Geometry: final body of the model. Coordinates: model frame, mm. Face numbers are marked on the shaded views. A direction names the side the tool comes from. Give positions to 0.01 mm unless a question says otherwise; leave off trailing zeros. Order: outer loops, then holes, each group sorted by start corner. A loop starts at its lowest first (then second) coordinate and runs counter-clockwise, first axis right, second up. Notation, with made-up numbers: M 10.25,37.5 L 20.25,37.5 A16 cw 20.25,41.5 Z; hole C 53.25,-34 d6. An arc over 180 degrees is marked long. Use CSV: the item, a comma, the result in double quotes.
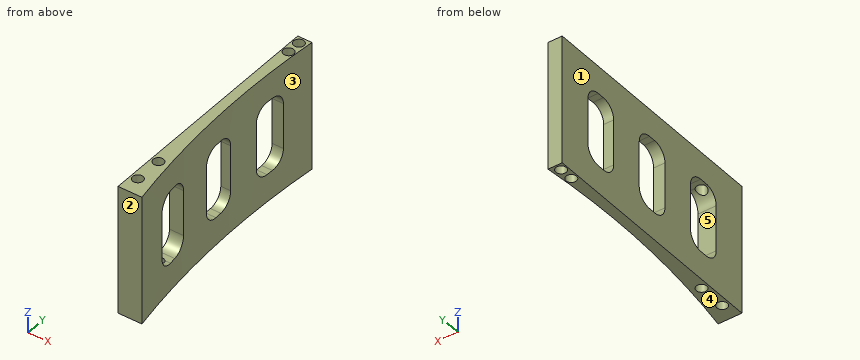
```python
from build123d import *

# Parameters (mm, degrees)
RESSALTO_EXTRUS_O1_DEPTH = 37.2
FILETE3_R                = 10
FILETE4_R                = 10
ESBO_O3_W                = 64.493903811
ESBO_O3_H                = 22.028162523
CORTE_EXTRUS_O2_DEPTH    = 126.622328301
ESBO_O4_W                = 56.697594262
ESBO_O4_H                = 123.119514717
CORTE_EXTRUS_O6_DEPTH    = 126.622328159
ESBO_O7_W                = 25.761955102
ESBO_O7_H                = 34.830585193
CORTE_EXTRUS_O7_DEPTH    = 125.245881598
CORTE_EXTRUS_O8_DEPTH    = 90.772656751
ESBO_O9_R                = 1.5
CORTE_EXTRUS_O9_DEPTH    = 92.227960203


with BuildPart() as part:
    # Esboço1 → Ressalto-extrusão1 (new body)
    with BuildSketch(Plane.XY):
        with BuildLine():
            ThreePointArc((-10, 0), (0, -10), (10, 0))
            Line((10, 0), (20, 0))
            ThreePointArc((20, 0), (14.071698091, 40.495175194), (14.829943665, 81.414963086))
            ThreePointArc((14.829943665, 81.414963086), (11.193742071, 116.066691762), (-16.576524471, 95.024435265))
            Line((-16.576524471, 95.024435265), (-16.487894969, 94.437265709))
            Line((-16.487894969, 94.437265709), (-16.369382775, 93.652123615))
            ThreePointArc((-16.369382775, 93.652123615), (-13.756795166, 46.654405302), (-20, 0))
            Line((-20, 0), (-10, 0))
        make_face()
    extrude(amount=RESSALTO_EXTRUS_O1_DEPTH)

    # Filete3
    # the kernel refuses this fillet: 10 mm, written as the material it takes off along each edge
    with BuildSketch(Plane(origin=(20, 0, -29.463728433), x_dir=(-0.20232831186330175, 0.9793177493635794, 0), z_dir=(0, 0, 1))) as filete3_piece_1:
        with BuildLine():
            CenterArc((12.021201201, 9.997221658), FILETE3_R, 181.169168083, 87.480189)
            Line((2.023283119, 9.793177494), (1.823324757, 9.78909661))
            ThreePointArc((1.823324757, 9.78909661), (0.815778009, 4.937054409), (-0.19586355, 0.040465662))
            Line((-0.19586355, 0.040465662), (0.004714197, -0.199944433))
            ThreePointArc((0.004714197, -0.199944433), (5.892745687, -0.130541448), (11.780777177, -0.199944433))
            Line((11.780777177, -0.199944433), (11.785491373, 0))
        make_face()
    extrude(amount=96.127456867, mode=Mode.SUBTRACT)
    with BuildSketch(Plane(origin=(-20, 0, -29.463728433), x_dir=(1, 0, 0), z_dir=(0, 0, 1))) as filete3_piece_2:
        with BuildLine():
            CenterArc((12.222685959, 9.749854723), FILETE3_R, 169.67749742, 87.480189)
            Line((2.384538574, 11.541740887), (2.187775626, 11.57757861))
            ThreePointArc((2.187775626, 11.57757861), (1.06442773, 5.797282674), (-0.194855317, 0.045071116))
            Line((-0.194855317, 0.045071116), (0, -0.2))
            ThreePointArc((0, -0.2), (5, -0.2), (9.955546281, -0.194997094))
            Line((9.955546281, -0.194997094), (10, 0))
        make_face()
    extrude(amount=96.127456867, mode=Mode.SUBTRACT)

    # Filete4
    filete4_edges = [part.edges().sort_by_distance(p)[0] for p in [
        (10, 0, 18.6),
        (-10, 0, 18.6),
    ]]
    fillet(filete4_edges, radius=FILETE4_R)

    # Esboço3 → Corte-extrusão2 (cut, through all)
    with BuildSketch(Plane.XY.offset(37.2)):
        with Locations((-2.119172362, 0.527659626)):
            Rectangle(ESBO_O3_W, ESBO_O3_H)
    extrude(amount=-CORTE_EXTRUS_O2_DEPTH, mode=Mode.SUBTRACT)

    # Esboço4 → Corte-extrusão6 (cut, through all)
    with BuildSketch(Plane.XY.offset(37.2)):
        with Locations((-17.581232159, 73.101498246)):
            Rectangle(ESBO_O4_W, ESBO_O4_H)
    extrude(amount=-CORTE_EXTRUS_O6_DEPTH, mode=Mode.SUBTRACT)

    # Esboço7 → Corte-extrusão7 (cut, through all)
    with BuildSketch(Plane.XY.offset(37.2)):
        with Locations((23.648542523, 98.830255682)):
            Rectangle(ESBO_O7_W, ESBO_O7_H)
    extrude(amount=-CORTE_EXTRUS_O7_DEPTH, mode=Mode.SUBTRACT)

    # Esboço8 → Corte-extrusão8 (cut, through all)
    with BuildSketch(Plane.ZY.offset(-10.767564972)):
        with BuildLine():
            Line((12, 71.414963086), (25.2, 71.414963086))
            ThreePointArc((25.2, 71.414963086), (28.028427125, 70.243390211), (29.2, 67.414963086))
            Line((29.2, 67.414963086), (29.2, 65.414963086))
            ThreePointArc((29.2, 65.414963086), (28.028427125, 62.586535961), (25.2, 61.414963086))
            Line((25.2, 61.414963086), (12, 61.414963086))
            ThreePointArc((12, 61.414963086), (9.171572875, 62.586535961), (8, 65.414963086))
            Line((8, 65.414963086), (8, 67.414963086))
            ThreePointArc((8, 67.414963086), (9.171572875, 70.243390211), (12, 71.414963086))
        make_face()
        with BuildLine():
            Line((12, 51.474963086), (25.2, 51.474963086))
            ThreePointArc((25.2, 51.474963086), (28.028427125, 50.303390211), (29.2, 47.474963086))
            Line((29.2, 47.474963086), (29.2, 45.474963086))
            ThreePointArc((29.2, 45.474963086), (28.028427125, 42.646535961), (25.2, 41.474963086))
            Line((25.2, 41.474963086), (12, 41.474963086))
            ThreePointArc((12, 41.474963086), (9.171572875, 42.646535961), (8, 45.474963086))
            Line((8, 45.474963086), (8, 47.474963086))
            ThreePointArc((8, 47.474963086), (9.171572875, 50.303390211), (12, 51.474963086))
        make_face()
        with BuildLine():
            Line((12, 31.541740887), (25.2, 31.541740887))
            ThreePointArc((25.2, 31.541740887), (28.028427125, 30.370168012), (29.2, 27.541740887))
            Line((29.2, 27.541740887), (29.2, 25.541740887))
            ThreePointArc((29.2, 25.541740887), (28.028427125, 22.713313762), (25.2, 21.541740887))
            Line((25.2, 21.541740887), (12, 21.541740887))
            ThreePointArc((12, 21.541740887), (9.171572875, 22.713313762), (8, 25.541740887))
            Line((8, 25.541740887), (8, 27.541740887))
            ThreePointArc((8, 27.541740887), (9.171572875, 30.370168012), (12, 31.541740887))
        make_face()
    extrude(amount=-CORTE_EXTRUS_O8_DEPTH, mode=Mode.SUBTRACT)

    # Esboço9 → Corte-extrusão9 (cut, through all)
    with BuildSketch(Plane(origin=(0, 0, 0), x_dir=(-1, 0, 0), z_dir=(0, 0, -1))):
        with Locations((-12.767564972, 16.541740887)):
            Circle(ESBO_O9_R)
        with Locations((-12.767564972, 24.541740887)):
            Circle(ESBO_O9_R)
        with Locations((-12.567564972, 79.414963086)):
            Circle(ESBO_O9_R)
        with Locations((-12.567564972, 75.414963086)):
            Circle(ESBO_O9_R)
    extrude(amount=-CORTE_EXTRUS_O9_DEPTH, mode=Mode.SUBTRACT)


solid = part.part
```
1. Pull-direction query (Y, two-part tool) for the marked faces 1, 2 and 3; classes: +Y half, -Y half, draft (parallel to the pull), parting line (faces both ways), or undercut.
Answer:
face 1,"draft"
face 2,"-Y half"
face 3,"undercut"
2. Reachability of the marked faces 4 and 5 from +Z, -Z, +X, -X, +Y, -Y: full face, straight path, thin tool, end or side. Return the list, or none.
Answer:
face 4,"-Z, +X, -X, +Y, -Y"
face 5,"+X, -X"
3. Section A-A, the plane z = 17. Return the cut outline in (x, y).
Answer:
outline,"M 10.77,11.54 L 17.62,11.54 A250 cw 16,21.54 L 10.77,21.54 Z; M 10.77,31.54 L 14.8,31.54 A250 cw 14.01,41.47 L 10.77,41.47 Z; M 10.77,51.47 L 13.62,51.47 A250 cw 13.62,61.41 L 10.77,61.41 Z; M 10.77,71.41 L 14.02,71.41 A250 cw 14.83,81.41 L 10.77,81.41 Z; hole C 12.57,75.41 d3; hole C 12.57,79.41 d3; hole C 12.77,16.54 d3"
4. Section B-B, the plane z = 32.5. Return the cut outline in (x, y), plus the area to 3 significant figures.
Answer:
outline,"M 10.77,11.54 L 17.62,11.54 A250 cw 14.83,81.41 L 10.77,81.41 Z; hole C 12.57,75.41 d3; hole C 12.57,79.41 d3; hole C 12.77,16.54 d3; hole C 12.77,24.54 d3"
area,"238 mm2"
5. Section D-D, the plane y = 59. Return the cut outline in (x, z).
Answer:
outline,"M 10.77,0 L 13.58,0 L 13.58,37.2 L 10.77,37.2 Z"
6. Pin query (flat end, axial travel): pin 1 Ø8 at (y, z) = (23, 28.5) entering from +X; pin 2 Ø5 at (y, z) = (55, 13) entering from +X; pin 3 Ø10 at (y, z) = (28.5, 22) entering from +X. Return the tip coordinate at first contact, or that it passes through.
Answer:
pin 1,"x = 16.37"
pin 2,"x = 13.6"
pin 3,"x = 14.81"
7. Line query: line 1 (Y direction, x = 12, z = 4.5); line 2 (Y direction, x = 12.5, z = 7); line 3 (X direction, y = 65, z = 6). Output: solid intervals per line, ascending.
Answer:
line 1,"11.54 to 15.25, 17.83 to 23.25, 25.83 to 74.03, 76.8 to 78.03, 80.8 to 81.41"
line 2,"11.54 to 15.07, 18.02 to 23.07, 26.02 to 73.92, 76.91 to 77.92, 80.91 to 81.41"
line 3,"10.77 to 13.72"
8. Section C-C, the plane z = 26.5. Return the cut outline in (x, y).
Answer:
outline,"M 10.77,11.54 L 17.62,11.54 A250 cw 15.97,21.76 L 10.77,21.76 Z; M 10.77,31.32 L 14.82,31.32 A250 cw 14,41.69 L 10.77,41.69 Z; M 10.77,51.26 L 13.62,51.26 A250 cw 13.63,61.63 L 10.77,61.63 Z; M 10.77,71.2 L 14.01,71.2 A250 cw 14.83,81.41 L 10.77,81.41 Z; hole C 12.57,75.41 d3; hole C 12.57,79.41 d3; hole C 12.77,16.54 d3"
